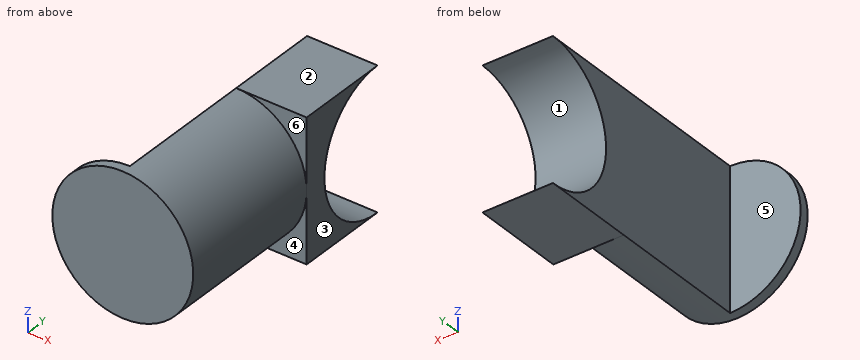
```python
from build123d import *

# Parameters (mm, degrees)
SKETCH1_R           = 75
BOSS_EXTRUDE1_DEPTH = 10
BOSS_EXTRUDE5_DEPTH = 150
SKETCH13_W          = 75
SKETCH13_H          = 150
BOSS_EXTRUDE6_DEPTH = 100
SKETCH14_R          = 75
CUT_EXTRUDE5_DEPTH  = 100


with BuildPart() as part:
    # Sketch1 → Boss-Extrude1 (new body)
    with BuildSketch(Plane(origin=(0, 0, 0), x_dir=(1, 0, 0), z_dir=(0, 1, 0))):
        with Locations(Location((0, 0, 0), (0, 0, 270))):
            Circle(SKETCH1_R)
    extrude(amount=BOSS_EXTRUDE1_DEPTH)

    # Sketch12 → Boss-Extrude5 (add)
    with BuildSketch(Plane(origin=(0, 10, 0), x_dir=(1, 0, 0), z_dir=(0, 1, 0))):
        with BuildLine():
            Line((0, 75), (0, -75))
            ThreePointArc((0, -75), (75, 0), (0, 75))
        make_face()
    extrude(amount=BOSS_EXTRUDE5_DEPTH)

    # Sketch13 → Boss-Extrude6 (add)
    with BuildSketch(Plane(origin=(0, 160, 0), x_dir=(1, 0, 0), z_dir=(0, 1, 0))):
        with Locations((37.5, 0)):
            Rectangle(SKETCH13_W, SKETCH13_H)
    extrude(amount=BOSS_EXTRUDE6_DEPTH)

    # Sketch14 → Cut-Extrude5 (cut)
    with BuildSketch(Plane.ZY):
        with Locations((0, 260)):
            Circle(SKETCH14_R)
    extrude(amount=-CUT_EXTRUDE5_DEPTH, mode=Mode.SUBTRACT)


solid = part.part
```
For this review, take the finished solid that the model builds, in its own axes (mm). Face numbers are marked on the shaded views. A direction names the side the tool comes from. Round coordinates to 2 decimals unless told otherwise and drop trailing zeros. Write each loop counter-clockwise with the first axis right and the second up, starting at its lowest first coordinate (ties: lowest second). Pieces come first, ordered by that corner, then holes. Notation, with made-up numbers: (-21, 40) - (13, 40) arc R6 ccw to (13, 46) - close; hole circle Ø5 at (-10.75, 23). An arc over 180 degrees is marked (long way). Answer as a JSON object with one key per item and string values.
1. To check wall thickness, follow line 1 along Y through (x, z) = (-14.5, -5); line 2 along X through (y, z) = (174, 45); line 3 along Z through (x, y) = (13, 204.5). State the ranges of each line that lie inside material, in increasing order.
Response values:
{"line 1": "y = 0 to 10", "line 2": "x = 0 to 75", "line 3": "z = -75 to -50.45, 50.45 to 75"}
2. We need section A-A on z = -37. Give the boundary of the cut face in (x, y), then the cut area to 3 significant figures.
Response values:
{"outline": "(-65.24, 0) - (65.24, 0) - (65.24, 160) - (75, 160) - (75, 194.76) - (0, 194.76) - (0, 10) - (-65.24, 10) - close", "area": "13,700 mm2"}
3. We need section D-D on x = -21. Give the boundary of the cut face in (y, z), then the cut area to 3 significant figures.
Response values:
{"outline": "(0, -72) - (10, -72) - (10, 72) - (0, 72) - close", "area": "1,440 mm2"}
4. Tool access review of the marked faces 4, 5 and 6: name each direction out of +Z, -Z, +X, -X, +Y, -Y from which nothing blocks a thin tool from reaching the whole face with its end or side.
Response values:
{"face 4": "-Z, +X, -Y", "face 5": "+Z, -Z, -X, +Y", "face 6": "+Z, +X, -Y"}
5. We need section C-C on y = 164. Give the boundary of the cut face in (x, z), then the cut area to 4 significant figures.
Response values:
{"outline": "(0, -75) - (75, -75) - (75, 75) - (0, 75) - close", "area": "11,250 mm2"}
6. We need section B-B on x = 39. Give the boundary of the cut face in (y, z), then the cut area to 3 significant figures.
Response values:
{"outline": "(0, -64.06) - (160, -64.06) - (160, -75) - (260, -75) arc R75 cw to (260, 75) - (160, 75) - (160, 64.06) - (0, 64.06) - close", "area": "26,700 mm2"}
7. Draft analysis for pull direction Z (two halves, no side actions). For the marked faces 1, 2 and 3, state which applies: +Z half, -Z half, draft (parallel to the pull), parting line (faces both ways), or undercut.
Response values:
{"face 1": "undercut", "face 2": "+Z half", "face 3": "draft"}
8. For pin 1 Ø12 at (y, z) = (61, -55) entering from +X; pin 2 Ø5 at (y, z) = (140, -26) entering from +X; pin 3 Ø12 at (x, z) = (26.5, 22) entering from +Y; pin 4 Ø22.5 at (x, z) = (26, -26.5) entering from -Y, all flat-tipped, find the tip position at first contact; note any pin that passes through.
Response values:
{"pin 1": "stops at x = 56.78", "pin 2": "stops at x = 71.22", "pin 3": "stops at y = 190.42", "pin 4": "stops at y = 0"}
